Geometry check sheet. Reference: drawing and pictorial views, mm from the part's lowest x, y, z. A direction names the side the tool comes from. Coordinates: 2 decimals unless noted, no trailing zeros. Write each loop counter-clockwise with the first axis right and the second up, starting at its lowest first coordinate (ties: lowest second). Pieces come first, ordered by that corner, then holes.
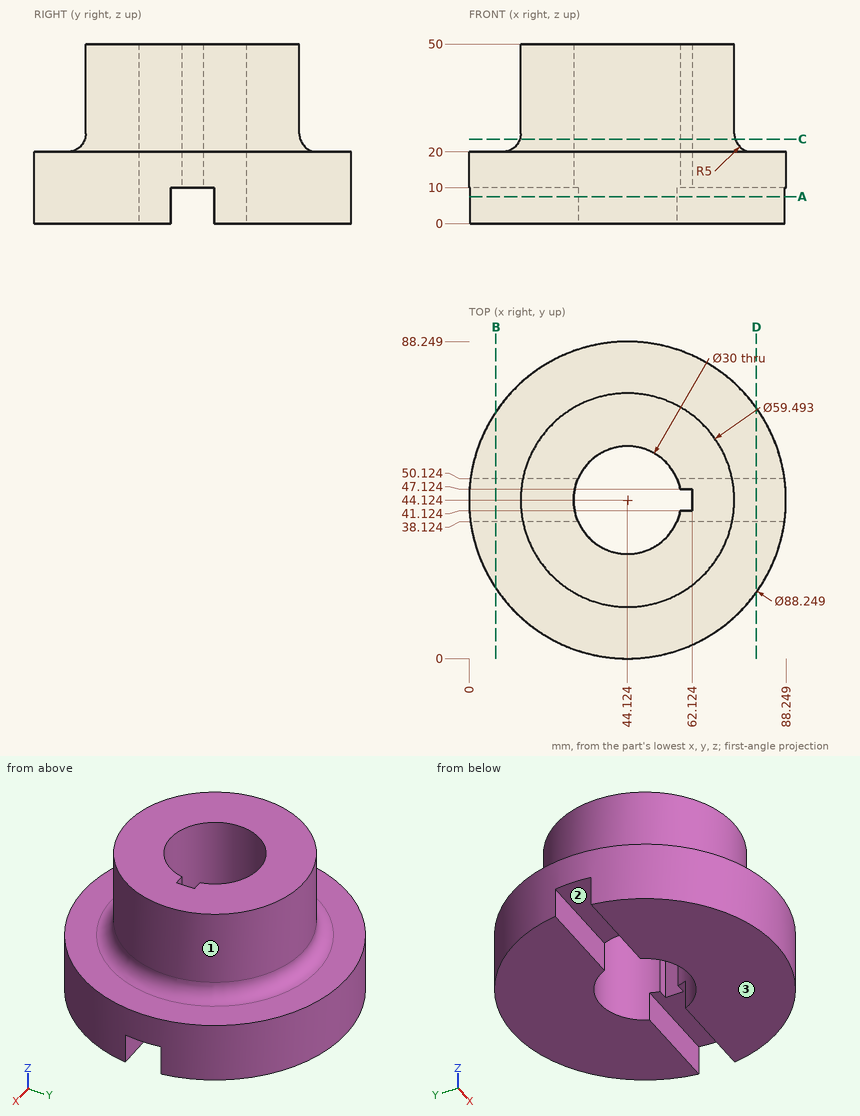
1. Material ranges on L1, parallel to Z at x = 73.5, y = 25.5; L2, parallel to X at y = 47, z = 35 (1 decimal); L3, parallel to Z at x = 7.5, y = 42, recorded low to high.
2. Sectioned sample at C-C, the plane z = 23.5. Record the boundary of the cut face in (x, y) (1 decimal).
3. Sectioned sample at A-A, the plane z = 7.5. Record the boundary of the cut face in (x, y) (1 decimal).
4. Sectioned sample at B-B, the plane x = 7.5. Record the boundary of the cut face in (y, z) (1 decimal).
5. Sectioned sample at D-D, the plane x = 80. Record the boundary of the cut face in (y, z) (1 decimal).
6. Gauge pin test, flat ends, axial feed: P1, Ø5, axis at x = 67.5, z = 20, coming from the +Y side; P2, Ø5, axis at x = 72.5, z = 3, coming from the -Y side; P3, Ø1.8, axis at y = 44.5, z = 32, coming from the -X side. Record the tip position at first contact, or that the pin passes through.
7. Tool access check on the marked faces 1, 2 and 3. Record the directions out of +Z, -Z, +X, -X, +Y, -Y that give a thin tool (end or side, any length) a straight path to the whole face; none if there is none.
Outcome:
1. L1: z = 0 to 20
1. L2: x = 14.5 to 29.4, 62.1 to 73.7
1. L3: z = 10 to 20
2. outline: circle Ø60 at (44.1, 44.1); hole (58.8, 41.1) - (62.1, 41.1) - (62.1, 47.1) - (58.8, 47.1) arc R15 ccw (long way) to start
3. outline: (0.4, 38.1) arc R44.1 ccw to (87.8, 38.1) - (57.9, 38.1) arc R15 cw to (30.4, 38.1) - close; (0.4, 50.1) - (30.4, 50.1) arc R15 cw to (57.9, 50.1) - (87.8, 50.1) arc R44.1 ccw to start
4. outline: (19.5, 0) - (38.1, 0) - (38.1, 10) - (50.1, 10) - (50.1, 0) - (68.7, 0) - (68.7, 20) - (19.5, 20) - close
5. outline: (18.4, 0) - (38.1, 0) - (38.1, 10) - (50.1, 10) - (50.1, 0) - (69.8, 0) - (69.8, 20) - (18.4, 20) - close
6. P1: stops at y = 83
6. P2: stops at y = 8.38
6. P3: stops at x = 14.38
7. face 1: +Z
7. face 2: -Z, +X, -X
7. face 3: -Z, +X, -X, +Y, -Y
